from build123d import *

# Parameters (mm, degrees)
BASE_FLANGE1_DEPTH         = 3.175
SKETCHED_START             = -150
SKETCHED_BEND1_DEPTH       = 300
SKETCHED_BEND1_2_DEPTH     = 70
SKETCHED_START_2           = 80
SKETCHED_BEND1_3_DEPTH     = 70
SKETCHED_BEND1_4_OUTLINE_W = 3.175
SKETCHED_BEND1_4_OUTLINE_H = 50
SKETCHED_BEND1_4_DEPTH     = 300
SKETCHED_START_3           = -80
SKETCHED_BEND1_5_DEPTH     = 160
SKETCH7_R                  = 4.815
CUT_EXTRUDE1_DEPTH         = 10
SKETCH8_R                  = 5
SKETCH8_R_2                = 1.025
CUT_EXTRUDE2_DEPTH         = 10
SKETCH9_R                  = 4.65
SKETCH9_R_2                = 5
SKETCH9_R_3                = 1.025
CUT_EXTRUDE3_DEPTH         = 10
CUT_EXTRUDE4_DEPTH         = 175.553238655
CUT_EXTRUDE5_DEPTH         = 175.553238655
SKETCH13_W                 = 30
SKETCH13_H                 = 100
CUT_EXTRUDE6_DEPTH         = 10
SKETCH14_W                 = 150
SKETCH14_H                 = 20
CUT_EXTRUDE7_DEPTH         = 175.553238655


# Read off the part's stored shape, not the designer's step: Sketched Bend1
# Sheet-metal steps are written as plain solids
with BuildPart() as part:
    # Sketch1 → Base-Flange1 (new body)
    with BuildSketch(Plane(origin=(0, 0, 0), x_dir=(1, 0, 0), z_dir=(0, 1, 0))):
        Polygon((-82.3, 150), (-32.3, 150), (-32.3, 80), (32.3, 80), (32.3, 150), (82.3, 150), (82.3, -150), (32.3, -150), (32.3, -80), (-32.3, -80), (-32.3, -150), (-82.3, -150), align=None)
    extrude(amount=-BASE_FLANGE1_DEPTH)

    # Sketched Bend1 outline → Sketched Bend1 (cut)
    with BuildSketch(Plane.XY.offset(SKETCHED_START)):
        with BuildLine():
            Line((-82.3, -3.175), (-35.353470735, -3.175))
            ThreePointArc((-35.353470735, -3.175), (-33.874453825, -0.888236775), (-31.3, 0))
            Line((-31.3, 0), (-82.3, 0))
            Line((-82.3, 0), (-82.3, -3.175))
        make_face()
        with BuildLine():
            Line((82.3, 0), (31.3, 0))
            ThreePointArc((31.3, 0), (33.874453825, -0.888236775), (35.353470735, -3.175))
            Line((35.353470735, -3.175), (82.3, -3.175))
            Line((82.3, -3.175), (82.3, 0))
        make_face()
    extrude(amount=SKETCHED_BEND1_DEPTH, mode=Mode.SUBTRACT)

    # Sketched Bend1 2 outline → Sketched Bend1 2 (cut)
    with BuildSketch(Plane.XY.offset(SKETCHED_START)):
        with BuildLine():
            Line((-35.353470735, -3.175), (-32.3, -3.175))
            Line((-32.3, -3.175), (-32.3, -0.121529265))
            ThreePointArc((-32.3, -0.121529265), (-34.252170811, -1.222829189), (-35.353470735, -3.175))
        make_face()
        with BuildLine():
            Line((32.3, -0.121529265), (32.3, -3.175))
            Line((32.3, -3.175), (35.353470735, -3.175))
            ThreePointArc((35.353470735, -3.175), (34.252170811, -1.222829189), (32.3, -0.121529265))
        make_face()
    extrude(amount=SKETCHED_BEND1_2_DEPTH, mode=Mode.SUBTRACT)

    # Sketched Bend1 3 outline → Sketched Bend1 3 (cut)
    with BuildSketch(Plane.XY.offset(SKETCHED_START_2)):
        with BuildLine():
            Line((-35.353470735, -3.175), (-32.3, -3.175))
            Line((-32.3, -3.175), (-32.3, -0.121529265))
            ThreePointArc((-32.3, -0.121529265), (-34.252170811, -1.222829189), (-35.353470735, -3.175))
        make_face()
        with BuildLine():
            Line((32.3, -0.121529265), (32.3, -3.175))
            Line((32.3, -3.175), (35.353470735, -3.175))
            ThreePointArc((35.353470735, -3.175), (34.252170811, -1.222829189), (32.3, -0.121529265))
        make_face()
    extrude(amount=SKETCHED_BEND1_3_DEPTH, mode=Mode.SUBTRACT)



with BuildPart() as body_2:
    # Sketched Bend1 4 outline → Sketched Bend1 4 (new body)
    with BuildSketch(Plane.XY.offset(SKETCHED_START)):
        with Locations((-33.8875, -29.175)):
            Rectangle(SKETCHED_BEND1_4_OUTLINE_W, SKETCHED_BEND1_4_OUTLINE_H)
        with Locations((33.8875, -29.175)):
            Rectangle(SKETCHED_BEND1_4_OUTLINE_W, SKETCHED_BEND1_4_OUTLINE_H)
    extrude(amount=SKETCHED_BEND1_4_DEPTH)


with BuildPart() as part_1:
    add(part.part)

    add(body_2.part)  # Sketched Bend1 5 merges body 2
    # Sketched Bend1 5 outline → Sketched Bend1 5 (add)
    with BuildSketch(Plane.XY.offset(SKETCHED_START_3)):
        with BuildLine():
            Line((-35.475, -4.175), (-32.3, -4.175))
            ThreePointArc((-32.3, -4.175), (-32.007106781, -3.467893219), (-31.3, -3.175))
            Line((-31.3, -3.175), (-35.353470735, -3.175))
            ThreePointArc((-35.353470735, -3.175), (-35.444506323, -3.671321193), (-35.475, -4.175))
        make_face()
        with BuildLine():
            Line((35.353470735, -3.175), (31.3, -3.175))
            ThreePointArc((31.3, -3.175), (32.007106781, -3.467893219), (32.3, -4.175))
            Line((32.3, -4.175), (35.475, -4.175))
            ThreePointArc((35.475, -4.175), (35.444506323, -3.671321193), (35.353470735, -3.175))
        make_face()
    extrude(amount=SKETCHED_BEND1_5_DEPTH)

    # Sketch7 → Cut-Extrude1 (cut)
    with BuildSketch(Plane(origin=(35.475, 0, 0), x_dir=(0, 0, -1), z_dir=(1, 0, 0))):
        with Locations(Location((-125, -29.175, 0), (0, 0, 90))):
            Circle(SKETCH7_R)
    extrude(amount=-CUT_EXTRUDE1_DEPTH, mode=Mode.SUBTRACT)

    # Sketch8 → Cut-Extrude2 (cut)
    with BuildSketch(Plane(origin=(35.475, 0, 0), x_dir=(0, 0, -1), z_dir=(1, 0, 0))):
        with Locations(Location((125, -29.175, 0), (0, 0, 90))):
            Circle(SKETCH8_R)
        with Locations(Location((125, -18.175, 0), (0, 0, 90))):
            Circle(SKETCH8_R_2)
        with Locations(Location((125, -40.175, 0), (0, 0, 90))):
            Circle(SKETCH8_R_2)
        with Locations(Location((136, -29.175, 0), (0, 0, 90))):
            Circle(SKETCH8_R_2)
        with Locations(Location((114, -29.175, 0), (0, 0, 90))):
            Circle(SKETCH8_R_2)
    extrude(amount=-CUT_EXTRUDE2_DEPTH, mode=Mode.SUBTRACT)

    # Sketch9 → Cut-Extrude3 (cut)
    with BuildSketch(Plane.ZY.offset(35.475)):
        with Locations(Location((-125, -29.175, 0), (0, 0, 270))):
            Circle(SKETCH9_R)
        with Locations(Location((125, -29.175, 0), (0, 0, 270))):
            Circle(SKETCH9_R_2)
        with Locations(Location((125, -18.175, 0), (0, 0, 270))):
            Circle(SKETCH9_R_3)
        with Locations(Location((114, -29.175, 0), (0, 0, 270))):
            Circle(SKETCH9_R_3)
        with Locations(Location((125, -40.175, 0), (0, 0, 270))):
            Circle(SKETCH9_R_3)
        with Locations(Location((136, -29.175, 0), (0, 0, 270))):
            Circle(SKETCH9_R_3)
    extrude(amount=-CUT_EXTRUDE3_DEPTH, mode=Mode.SUBTRACT)

    # Sketch10 → Cut-Extrude4 (cut, through all)
    with BuildSketch(Plane(origin=(35.475, 0, 0), x_dir=(0, 0, -1), z_dir=(1, 0, 0))):
        with BuildLine():
            ThreePointArc((-150, -29.175), (-142.67766953, -11.49733047), (-125, -4.175))
            Line((-125, -4.175), (-150, -4.175))
            Line((-150, -4.175), (-150, -29.175))
        make_face()
        with BuildLine():
            ThreePointArc((-125, -54.175), (-142.67766953, -46.85266953), (-150, -29.175))
            Line((-150, -29.175), (-150, -54.175))
            Line((-150, -54.175), (-125, -54.175))
        make_face()
    extrude(amount=-CUT_EXTRUDE4_DEPTH, mode=Mode.SUBTRACT)

    # Sketch11 → Cut-Extrude5 (cut, through all)
    with BuildSketch(Plane(origin=(35.475, 0, 0), x_dir=(0, 0, -1), z_dir=(1, 0, 0))):
        with BuildLine():
            Line((150, -4.175), (125, -4.175))
            ThreePointArc((125, -4.175), (142.67766953, -11.49733047), (150, -29.175))
            Line((150, -29.175), (150, -4.175))
        make_face()
        with BuildLine():
            Line((150, -54.175), (150, -29.175))
            ThreePointArc((150, -29.175), (142.67766953, -46.85266953), (125, -54.175))
            Line((125, -54.175), (150, -54.175))
        make_face()
    extrude(amount=-CUT_EXTRUDE5_DEPTH, mode=Mode.SUBTRACT)

    # Sketch13 → Cut-Extrude6 (cut)
    with BuildSketch(Plane(origin=(0, 0, 0), x_dir=(1, 0, 0), z_dir=(0, 1, 0))):
        Rectangle(SKETCH13_W, SKETCH13_H)
    extrude(amount=-CUT_EXTRUDE6_DEPTH, mode=Mode.SUBTRACT)

    # Sketch14 → Cut-Extrude7 (cut, through all)
    with BuildSketch(Plane.ZY.offset(35.475)):
        with Locations((0, -29.175)):
            Rectangle(SKETCH14_W, SKETCH14_H)
    extrude(amount=-CUT_EXTRUDE7_DEPTH, mode=Mode.SUBTRACT)


solid = part_1.part
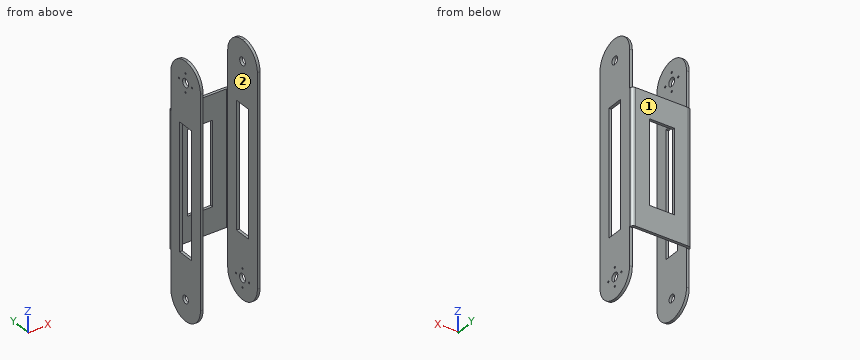
Input: part model. Units: mm. Frame: model coordinates. Face numbers are marked on the shaded views. A direction names the side the tool comes from. Coordinates: 2 decimals unless noted, no trailing zeros. Write each loop counter-clockwise with the first axis right and the second up, starting at its lowest first coordinate (ties: lowest second). Pieces come first, ordered by that corner, then holes. Notation, with made-up numbers: M 78,-14.5 L 108,-14.5 A28 ccw 108,15.5 Z; hole C 13.25,70 d2. An arc over 180 degrees is marked long. Answer as a JSON object with one key per item and string values. Group by question number.
(1) Section A-A on z = 56. Output: boundary loops of the cut face in (x, y) (3 decimals).
(2) Section B-B on x = -1.5. Output: boundary loops of the cut face in (y, z) (3 decimals), plus the area to 4 significant figures.
(3) Contact query for flat-ended pins moving along their axis: P1, Ø12, axis at x = 21.5, z = 53.5, coming from the -Y side (3 decimals); P2, Ø6, axis at y = -29.175, z = 125, coming from the -X side; P3, Ø1.3, axis at x = 5, y = -1.5, coming from the +Z side; P4, Ø1.6, axis at x = 34, z = -27, coming from the +Y side. Output: stop coordinate, or through.
(4) Section C-C on x = -26.5. Output: boundary loops of the cut face in (y, z) (3 decimals).
(5) Set-up query: the marked faces 1 and 2. Return all of +Z, -Z, +X, -X, +Y, -Y with unobstructed straight access to the full face (end or side cutting, diameter ignored); none if empty.
(6) Ray query, line 1 along X through (y, z) = (-6.5, -29.5) (3 decimals); line 2 along Y through (x, z) = (-34.35, 136); line 3 along Y through (x, z) = (-11.5, -71.5) (3 decimals). Return the intervals inside material, ascending. Write a range as [from, to].
Result set:
{
 "1": {"outline": "M -35.475,-54.175 L -32.3,-54.175 L -32.3,-39.175 L -35.475,-39.175 Z; M -35.475,-19.175 L -32.3,-19.175 L -32.3,-4.175 A1 cw -31.3,-3.175 L 31.3,-3.175 A1 cw 32.3,-4.175 L 32.3,-19.175 L 35.475,-19.175 L 35.475,-4.175 A4.175 ccw 31.3,0 L -31.3,0 A4.175 ccw -35.475,-4.175 Z; M 32.3,-54.175 L 35.475,-54.175 L 35.475,-39.175 L 32.3,-39.175 Z"},
 "2": {"outline": "M -3.175,-80 L 0,-80 L 0,-50 L -3.175,-50 Z; M -3.175,50 L 0,50 L 0,80 L -3.175,80 Z", "area": "190.5 mm2"},
 "3": {"P1": "stops at y = -3.175", "P2": "passes through", "P3": "stops at z = 80", "P4": "stops at y = -0.46"},
 "4": {"outline": "M -3.175,-80 L 0,-80 L 0,80 L -3.175,80 Z"},
 "5": {"face 1": "+Z, -Z, +X, -X, +Y", "face 2": "+Z, -Z, -Y"},
 "6": {"line 1": "x = [-35.475, -32.3], [32.3, 35.475]", "line 2": "y = [-51.62, -30.2], [-28.15, -6.73]", "line 3": "y = [-3.175, 0]"}
}
